from build123d import *

# Parameters (mm, degrees)
SKETCH1_W                      = 6
SKETCH1_H                      = 3.5
BASE_DEPTH                     = 0.5
TAB_DEPTH                      = 0.5
SKETCH3_R                      = 0.5
SOLDERING_HOLE_DEPTH           = 7.509608283
SKETCH4_R                      = 0.5
RIVET_HOLE_DEPTH               = 7.509608283
FIRST_START                    = -3
FIRST_SIDE_TAB_DEPTH           = 2.15
FIRST_SIDE_TAB_2_DEPTH         = 2
FIRST_START_2                  = -1
FIRST_SIDE_TAB_3_DEPTH         = 2.2
SECOND_ANGLED_SIDE_TAB_DEPTH   = 2
SECOND_START                   = 1.2
SECOND_ANGLED_SIDE_TAB_2_DEPTH = 0.8
THIRD_ANGLED_SIDE_TAB_DEPTH    = 2
MIRROR1_DEPTH                  = 0.5
MIRROR1_2_OUTLINE_W            = 2
MIRROR1_2_OUTLINE_H            = 0.5
MIRROR1_2_DEPTH                = 0.04719
MIRROR1_3_DEPTH                = 2
MIRROR1_START                  = 1.2
MIRROR1_4_DEPTH                = 0.8
MIRROR1_START_2                = -3
MIRROR1_5_DEPTH                = 2
MIRROR1_6_DEPTH                = 2


with BuildPart() as part:
    # Sketch1 → BASE (new body)
    with BuildSketch(Plane(origin=(0, 0, 0), x_dir=(1, 0, 0), z_dir=(0, 1, 0))):
        Rectangle(SKETCH1_W, SKETCH1_H)
    extrude(amount=BASE_DEPTH)

    # Sketch2 → TAB (add)
    with BuildSketch(Plane(origin=(0, 0, 0), x_dir=(1, 0, 0), z_dir=(0, 1, 0))):
        with BuildLine():
            Line((5, -1.25), (3, -1.25))
            ThreePointArc((3, -1.25), (1.75, 0), (3, 1.25))
            Line((3, 1.25), (5, 1.25))
            ThreePointArc((5, 1.25), (6.25, 0), (5, -1.25))
        make_face()
    extrude(amount=TAB_DEPTH)

    # Sketch3 → SOLDERING HOLE (cut, through all)
    with BuildSketch(Plane(origin=(0, 0.5, 0), x_dir=(1, 0, 0), z_dir=(0, 1, 0))):
        with Locations(Location((5, 0, 0), (0, 0, 270))):
            Circle(SKETCH3_R)
    extrude(amount=-SOLDERING_HOLE_DEPTH, mode=Mode.SUBTRACT)

    # Sketch4 → RIVET HOLE (cut, through all)
    with BuildSketch(Plane(origin=(0, 0.5, 0), x_dir=(1, 0, 0), z_dir=(0, 1, 0))):
        with Locations(Location((1, 0, 0), (0, 0, 270))):
            Circle(SKETCH4_R)
    extrude(amount=-RIVET_HOLE_DEPTH, mode=Mode.SUBTRACT)

    # FIRST SIDE TAB: read off the stored shape, not the designer's step
    # FIRST SIDE TAB outline → FIRST SIDE TAB (cut)
    with BuildSketch(Plane.YZ.offset(FIRST_START)):
        with BuildLine():
            ThreePointArc((0, 0.55), (0.132292175, 1.097722557), (0.5, 1.524679434))
            Line((0.5, 1.524679434), (0.5, 1.75))
            Line((0.5, 1.75), (0, 1.75))
            Line((0, 1.75), (0, 0.55))
        make_face()
    extrude(amount=FIRST_SIDE_TAB_DEPTH, mode=Mode.SUBTRACT)

    # FIRST SIDE TAB 2 outline → FIRST SIDE TAB 2 (add)
    with BuildSketch(Plane.YZ.offset(FIRST_START)):
        with BuildLine():
            Line((2, 1.75), (1.2, 1.75))
            ThreePointArc((1.2, 1.75), (0.832314891, 1.692281778), (0.5, 1.524679434))
            Line((0.5, 1.524679434), (0.5, 0.55))
            ThreePointArc((0.5, 0.55), (0.705025253, 1.044974747), (1.2, 1.25))
            Line((1.2, 1.25), (2, 1.25))
            Line((2, 1.25), (2, 1.75))
        make_face()
    extrude(amount=FIRST_SIDE_TAB_2_DEPTH)

    # FIRST SIDE TAB 3 outline → FIRST SIDE TAB 3 (cut)
    with BuildSketch(Plane(origin=(0, 0, 0), x_dir=(1, 0, 0), z_dir=(0, 1, 0)).offset(FIRST_START_2)):
        with BuildLine():
            Line((-0.85, -3), (-0.85, -0.4))
            ThreePointArc((-0.85, -0.4), (-0.925, -0.325), (-1, -0.4))
            Line((-1, -0.4), (-1, -3))
            Line((-1, -3), (-0.85, -3))
        make_face()
    extrude(amount=FIRST_SIDE_TAB_3_DEPTH, mode=Mode.SUBTRACT)



with BuildPart() as body_2:
    # SECOND ANGLED SIDE TAB: read off the stored shape, not the designer's step
    # SECOND ANGLED SIDE TAB outline → SECOND ANGLED SIDE TAB (new body)
    with BuildSketch(Plane(origin=(0, 0, 0), x_dir=(1, 0, 0), z_dir=(0, 1, 0))):
        Polygon((-6.113516821, -0.69378588), (-3.410424172, -1.677631145), (-3.2394141, -1.207784835), (-5.942506749, -0.22393957), align=None)
    extrude(amount=SECOND_ANGLED_SIDE_TAB_DEPTH)


with BuildPart() as part_1:
    add(part.part)

    add(body_2.part)  # SECOND ANGLED SIDE TAB 2 merges body 2
    # SECOND ANGLED SIDE TAB 2 outline → SECOND ANGLED SIDE TAB 2 (add)
    with BuildSketch(Plane(origin=(0, 0, 0), x_dir=(1, 0, 0), z_dir=(0, 1, 0)).offset(SECOND_START)):
        with BuildLine():
            Line((-3.2394141, -1.207784835), (-3.410424172, -1.677631145))
            ThreePointArc((-3.410424172, -1.677631145), (-3.208377813, -1.731769304), (-3, -1.75))
            Line((-3, -1.75), (-3, -1.25))
            ThreePointArc((-3, -1.25), (-3.121553724, -1.239365427), (-3.2394141, -1.207784835))
        make_face()
    extrude(amount=SECOND_ANGLED_SIDE_TAB_2_DEPTH)

    # THIRD ANGLED SIDE TAB: sheet metal written as solids
    # THIRD ANGLED SIDE TAB section (on a plane across the edge) → THIRD ANGLED SIDE TAB (add)
    with BuildSketch(Plane(origin=(-6.352930921, 2, 0.606646274), x_dir=(0.3420201433256691, 0, 0.9396926207859083), z_dir=(0, -1, 0))):
        with BuildLine():
            Line((-0.5, 0.254779164), (-0.5, 2))
            Line((-0.5, 2), (0, 2))
            Line((0, 2), (0, 0.254779164))
            ThreePointArc((0, 0.254779164), (0.042215165, 0.015365064), (0.16376889, -0.195172163))
            Line((0.16376889, -0.195172163), (-0.219253332, -0.516565968))
            ThreePointArc((-0.219253332, -0.516565968), (-0.427631145, -0.155645008), (-0.5, 0.254779164))
        make_face()
    extrude(amount=THIRD_ANGLED_SIDE_TAB_DEPTH)

    # Mirror1: read off the stored shape, not the designer's step
    # Mirror1 outline → Mirror1 (cut)
    with BuildSketch(Plane(origin=(0, 0, 0), x_dir=(1, 0, 0), z_dir=(0, 1, 0))):
        with BuildLine():
            Line((-0.85, 1.75), (-1, 1.75))
            Line((-1, 1.75), (-1, 0.4))
            ThreePointArc((-1, 0.4), (-0.925, 0.325), (-0.85, 0.4))
            Line((-0.85, 0.4), (-0.85, 1.75))
        make_face()
    extrude(amount=MIRROR1_DEPTH, mode=Mode.SUBTRACT)

    # Mirror1 2 outline → Mirror1 2 (cut)
    with BuildSketch(Plane(origin=(0, 0, 0), x_dir=(1, 0, 0), z_dir=(0, 1, 0))):
        with Locations((-2, 1.5)):
            Rectangle(MIRROR1_2_OUTLINE_W, MIRROR1_2_OUTLINE_H)
    extrude(amount=MIRROR1_2_DEPTH, mode=Mode.SUBTRACT)

    # Mirror1 5 outline → Mirror1 5 (cut)
    with BuildSketch(Plane.YZ.offset(MIRROR1_START_2)):
        with BuildLine():
            Line((0.5, -1.75), (0.5, -1.524679434))
            ThreePointArc((0.5, -1.524679434), (0.132292175, -1.097722557), (0, -0.55))
            Line((0, -0.55), (0, -1.25))
            Line((0, -1.25), (0.04719, -1.25))
            Line((0.04719, -1.25), (0.04719, -1.75))
            Line((0.04719, -1.75), (0.5, -1.75))
        make_face()
    extrude(amount=MIRROR1_5_DEPTH, mode=Mode.SUBTRACT)



with BuildPart() as body_2_2:
    # Mirror1 3 outline → Mirror1 3 (new body)
    with BuildSketch(Plane(origin=(0, 0, 0), x_dir=(1, 0, 0), z_dir=(0, 1, 0))):
        with BuildLine():
            Line((-3.2394141, 1.207784835), (-3.410424172, 1.677631145))
            Line((-3.410424172, 1.677631145), (-6.113516821, 0.69378588))
            ThreePointArc((-6.113516821, 0.69378588), (-6.352930921, 0.651570715), (-6.592345021, 0.69378588))
            Line((-6.592345021, 0.69378588), (-8.232316162, 1.290686561))
            Line((-8.232316162, 1.290686561), (-8.403326234, 0.82084025))
            Line((-8.403326234, 0.82084025), (-6.763355093, 0.22393957))
            ThreePointArc((-6.763355093, 0.22393957), (-6.352930921, 0.151570715), (-5.942506749, 0.22393957))
            Line((-5.942506749, 0.22393957), (-3.2394141, 1.207784835))
        make_face()
    extrude(amount=MIRROR1_3_DEPTH)

    # Mirror1 4 outline → Mirror1 4 (add)
    with BuildSketch(Plane(origin=(0, 0, 0), x_dir=(1, 0, 0), z_dir=(0, 1, 0)).offset(MIRROR1_START)):
        with BuildLine():
            Line((-1, 1.75), (-3, 1.75))
            ThreePointArc((-3, 1.75), (-3.208377813, 1.731769304), (-3.410424172, 1.677631145))
            Line((-3.410424172, 1.677631145), (-3.2394141, 1.207784835))
            ThreePointArc((-3.2394141, 1.207784835), (-3.121553724, 1.239365427), (-3, 1.25))
            Line((-3, 1.25), (-1, 1.25))
            Line((-1, 1.25), (-1, 1.75))
        make_face()
    extrude(amount=MIRROR1_4_DEPTH)


with BuildPart() as part_2:
    add(part_1.part)

    add(body_2_2.part)  # Mirror1 6 merges body 2 2
    # Mirror1 6 outline → Mirror1 6 (add)
    with BuildSketch(Plane.YZ.offset(MIRROR1_START_2)):
        with BuildLine():
            ThreePointArc((0.5, -1.524679434), (0.832314891, -1.692281778), (1.2, -1.75))
            Line((1.2, -1.75), (1.2, -1.25))
            ThreePointArc((1.2, -1.25), (0.705025253, -1.044974747), (0.5, -0.55))
            Line((0.5, -0.55), (0.5, -1.524679434))
        make_face()
    extrude(amount=MIRROR1_6_DEPTH)


solid = part_2.part
Geometry: final body of the model. Coordinates: model frame, mm. A direction names the side the tool comes from. Round coordinates to 2 decimals unless told otherwise and drop trailing zeros. Loops run counter-clockwise (first coordinate to the right, second up) from the corner with the lowest first, then second, coordinate; pieces in that order, holes last. Notation, with made-up numbers: M -36.5,-4.5 L -26.5,-4.5 A29 ccw -26.5,22.5 Z; hole C 24,-29 d3. An arc over 180 degrees is marked long. Put each result on its own line as item: value. Start each with the question number.
(1) Material intervals for line 1 along X through (y, z) = (0.15, 0); line 2 along Y through (x, z) = (2.5, 1.4); line 3 along Z through (x, y) = (-6.25, 0.5), sorted ascending. Write a range as [from, to].
(2) Section query A-A (y = 1.55). Return loops of the section in (x, z).
(3) Contact query for flat-ended pins moving along their axis: pin 1 Ø0.7 at (y, z) = (1, -1) entering from +X; pin 2 Ø1 at (y, z) = (0.5, 1.5) entering from +X; pin 3 Ø1 at (x, z) = (2.5, 0.5) entering from +Y. Output: stop coordinate, or through.
(4) Set-up query: faces 4 (the face through (-4.572, 0.986, 0.723)), 5 (the face through (6.25, 0.25, -0.03)), 6 (the face through (-1, 0.8, -1.4)), 7 (the face through (-7.595, 0.986, -0.527)). Return all of +Z, -Z, +X, -X, +Y, -Y with unobstructed straight access to the full face (end or side cutting, diameter ignored); none if empty.
(5) Draft query along Z for faces 1 (the face through (-6.36, 0.99, -0.15)), 2 (the face through (-1, 0.8, 1.4)), 3 (the face through (-4.78, 0.99, 1.18)). Return one class per face: +Z half, -Z half, draft (parallel to the pull), parting line (faces both ways), or undercut.
(6) Section query D-D (y = 0.2). State how many separate pieces and enclosed holes the cut face has, then the cut area to 3 significant figures.
(7) Section query C-C (z = 0). Return loops of the section in (x, y).
(8) Section query B-B (x = 1). Return loops of the section in (y, z).
Findings below:
1. line 1: x = [-3, 0.5], [1.5, 4.5], [5.5, 6.25]
1. line 2: y = [0, 0.5]
1. line 3: z = [-0.66, -0.16], [0.16, 0.66]
2. outline: M -8.4,-0.82 L -8.23,-1.29 L -6.59,-0.69 A0.7 cw -6.11,-0.69 L -3.41,-1.68 A1.2 ccw -3,-1.75 L -1,-1.75 L -1,-1.25 L -3,-1.25 A0.7 cw -3.24,-1.21 L -5.94,-0.22 A1.2 ccw -6.76,-0.22 Z; M -8.4,0.82 L -6.76,0.22 A1.2 ccw -5.94,0.22 L -3.24,1.21 A0.7 cw -3,1.25 L -1,1.25 L -1,1.75 L -3,1.75 A1.2 ccw -3.41,1.68 L -6.11,0.69 A0.7 cw -6.59,0.69 L -8.23,1.29 Z
3. pin 1: stops at x = -1
3. pin 2: stops at x = 5.75
3. pin 3: stops at y = 0.5
4. face 4: +Y, -Y
4. face 5: +X, +Y, -Y
4. face 6: -Z, +Y, -Y
4. face 7: -X, +Y, -Y
5. face 1: undercut
5. face 2: draft
5. face 3: +Z half
6. separate pieces: 3
6. enclosed holes: 2
6. area: 29.6 mm2
7. outline: M -3,0 L 0.5,0 L 0.5,0.5 L -3,0.5 Z; M 1.5,0 L 4.5,0 L 4.5,0.5 L 1.5,0.5 Z; M 5.5,0 L 6.25,0 L 6.25,0.5 L 5.5,0.5 Z
8. outline: M 0,-1.75 L 0.5,-1.75 L 0.5,-0.5 L 0,-0.5 Z; M 0,0.5 L 0.5,0.5 L 0.5,1.75 L 0,1.75 Z
